Check sheet for the modelled part. Datum: model origin and axes. Units: mm. Round coordinates to 2 decimals unless told otherwise and drop trailing zeros. Loops run counter-clockwise (first coordinate to the right, second up) from the corner with the lowest first, then second, coordinate; pieces in that order, holes last. Notation, with made-up numbers: (62, 17) - (68, 17) arc R17 ccw to (68, 33) - close; hole circle Ø9 at (4.25, 33.5). An arc over 180 degrees is marked (long way). Return JSON: item names as keys, results as strings.
Autodesk Inventor part; units mm, degrees
ref_plane "YZ Plane" through (0, 0, 0) normal (1, 0, 0) x (0, 1, 0)
ref_plane "XZ Plane" through (0, 0, 0) normal (0, 1, 0) x (-1, 0, 0)
ref_plane "XY Plane" through (0, 0, 0) normal (0, 0, 1) x (1, 0, 0)
sketch "Sketch2" plane through (0, 0, 0) normal (0, 1, 0) x (-1, 0, 0)
  line L0 (0, 0) -> (100, 0)
  line L1 (100, 0) -> (100, -100)
  line L2 (100, -100) -> (0, -100)
  line L3 (0, -100) -> (0, 0)
  circle A0 centre (82.5, -5) radius 1.75
  circle A1 centre (82.5, -95) radius 1.75
  circle A2 centre (17.5, -5) radius 1.75
  circle A3 centre (17.5, -95) radius 1.75
  circle A4 centre (80, -30) radius 1.75
  circle A5 centre (91.5, -21) radius 1.75
  circle A6 centre (91.5, -79) radius 1.75
  circle A7 centre (5.5, -21) radius 1.75
  circle A8 centre (5.5, -79) radius 1.75
  line L4 (50, 0) -> (50, -100)
  circle A9 centre (40, -30) radius 1.75
  circle A10 centre (80, -70) radius 1.75
  circle A11 centre (40, -70) radius 1.75
  dimension "d13" = 100
  dimension "d14" = 100
  dimension "d15" = 3.5
  dimension "d16" = 17.5
  dimension "d17" = 5
  dimension "d20" = 90
  dimension "d23" = 65
  dimension "d26" = 3.5
  dimension "d27" = 20
  dimension "d28" = 30
  dimension "d32" = 3.5
  dimension "d35" = 58
  dimension "d38" = 86
  dimension "d41" = 8.5
  dimension "d42" = 21
  dimension "d51" = 40
  dimension "d54" = 40
extrude "Extrusion2" add sketch "Sketch2" along normal blind 6
fillet "Fillet2" radius 5 4 edges at (0, 3, -100) (-100, 3, -100) (0, 3, 0) (-100, 3, 0)
sketch "Sketch3" plane through (0, 6, 0) normal (0, 1, 0) x (1, 0, 0)
  circle A0 centre (-74.5, 27) radius 2
  line L0 (-100, 95) -> (-100, 5)
  line L1 (-95, 0) -> (-5, 0)
  circle A1 centre (-25.5, 27) radius 2
  circle A2 centre (-74.5, 85) radius 2
  circle A3 centre (-25.5, 85) radius 2
  point P0 (0, 0)
  dimension "d57" = 4
  dimension "d58" = 25.5
  dimension "d59" = 27
  dimension "d62" = 49
  dimension "d65" = 58
extrude "Extrusion3" cut sketch "Sketch3" against normal through all
properties part number "EboxMounting_Plate"
Q1. Scan lines: probe 1 along X at (y, z) = (4.2, -70); probe 2 along X at (y, z) = (4.35, -27); probe 3 along Z at (x, y) = (-17.5, 2.1). Record each from-to range of solid material in increasing order. Write a range as [from, to].
Answer key:
{"probe 1": "x = [-100, -81.75], [-78.25, -41.75], [-38.25, 0]", "probe 2": "x = [-100, -76.5], [-72.5, -27.5], [-23.5, 0]", "probe 3": "z = [-100, -96.75], [-93.25, -6.75], [-3.25, 0]"}
Q2. Sectioned sample at C-C (y = 3.75). State how many separate pieces and enclosed holes the cut face has, plus the area to 3 significant figures.
Answer key:
{"separate pieces": "1", "enclosed holes": "16", "area": "9,810 mm²"}
Q3. Sectioned sample at B-B (z = -85). Enter the section's corners in (x, y).
Answer key:
{"outline": "(-100, 0) - (-76.5, 0) - (-76.5, 6) - (-100, 6) - close; (-72.5, 0) - (-27.5, 0) - (-27.5, 6) - (-72.5, 6) - close; (-23.5, 0) - (0, 0) - (0, 6) - (-23.5, 6) - close"}
Q4. Sectioned sample at A-A (x = -25.5). Enter the section's corners in (y, z), plus the area to 3 significant figures.
Answer key:
{"outline": "(0, -100) - (6, -100) - (6, -87) - (0, -87) - close; (0, -83) - (6, -83) - (6, -29) - (0, -29) - close; (0, -25) - (6, -25) - (6, 0) - (0, 0) - close", "area": "552 mm²"}
